Read the model definition and answer for the solid it produces. Units are mm, in the model's axes. A direction names the side the tool comes from. Round coordinates to 2 decimals unless told otherwise and drop trailing zeros. Loops run counter-clockwise (first coordinate to the right, second up) from the corner with the lowest first, then second, coordinate; pieces in that order, holes last. Notation, with made-up numbers: (-33.75, 3) - (-26.75, 3) arc R31 cw to (-26.75, 35) - close; hole circle Ø4 at (49.5, 5.25). An arc over 180 degrees is marked (long way). Use one line per item in the form item = value. Start each with the question number.
```python
from build123d import *

# Parameters (mm, degrees)
PAD028_DEPTH    = 1.4
SKETCH048_R     = 1.75
PAD029_DEPTH    = 1
PAD030_DEPTH    = 1
PAD031_DEPTH    = 1
SKETCH181_W     = 1.5
SKETCH181_H     = 1.5
POCKET062_DEPTH = 1


with BuildPart() as part:
    # Sketch047 (on Face725 of Binder021) → Pad028 (new body)
    with BuildSketch(Plane(origin=(0, 135.8, 0), x_dir=(-1, 0, 0), z_dir=(0, 1, 0))):
        with BuildLine():
            Line((-120.499982, -0.1), (-120.499982, -26.3))
            Line((-120.499982, -26.3), (-68.48194, -26.3))
            ThreePointArc((-67.46705, -26.3), (-67.974495, -21.15), (-68.48194, -26.3))
            Line((-67.46705, -26.3), (-32.299995, -26.3))
            Line((-32.299995, -15.934266), (-32.299995, -26.3))
            ThreePointArc((-31.615729, -15.25), (-32.099578, -15.450417), (-32.299995, -15.934266))
            Line((-31.615729, -15.25), (-23.784261, -15.25))
            ThreePointArc((-23.099995, -15.934266), (-23.300412, -15.450417), (-23.784261, -15.25))
            Line((-23.099995, -15.934266), (-23.099995, -26.3))
            Line((-7.299995, -26.3), (-23.099995, -26.3))
            Line((-7.299995, -26.3), (-7.299995, -0.1))
            Line((-7.299995, -0.1), (-120.499982, -0.1))
        make_face()
        with BuildLine():
            Line((-105.199995, -19.86), (-92.199994, -19.86))
            ThreePointArc((-90.899995, -21.16), (-91.280756, -20.240762), (-92.199994, -19.86))
            Line((-90.899995, -21.16), (-90.899995, -24.776619))
            Line((-90.899995, -24.776619), (-91.938732, -25.120886))
            Line((-91.938732, -25.120886), (-92.869018, -25.773985))
            ThreePointArc((-93.61597, -26.01), (-93.224294, -25.949593), (-92.869018, -25.773985))
            Line((-93.61597, -26.01), (-103.78402, -26.01))
            ThreePointArc((-104.530977, -25.773981), (-104.175699, -25.949592), (-103.78402, -26.01))
            Line((-105.461258, -25.120886), (-104.530977, -25.773981))
            Line((-106.499995, -24.776619), (-105.461258, -25.120886))
            Line((-106.499995, -21.16), (-106.499995, -24.776619))
            ThreePointArc((-105.199995, -19.86), (-106.119234, -20.240761), (-106.499995, -21.16))
        make_face(mode=Mode.SUBTRACT)
    extrude(amount=-PAD028_DEPTH)

    # Sketch048 (on Face5 of Binder022) → Pad029 (join)
    with BuildSketch(Plane.XY.offset(-26.3)):
        with BuildLine():
            Line((18.199995, 134.4), (8.199995, 134.4))
            Line((8.199995, 134.4), (8.199995, 124.1))
            Line((8.199995, 124.1), (13.199995, 124.1))
            ThreePointArc((13.199995, 124.1), (16.735529, 125.564466), (18.199995, 129.1))
            Line((18.199995, 134.4), (18.199995, 129.1))
        make_face()
        with Locations((13.199995, 129.1)):
            Circle(SKETCH048_R, mode=Mode.SUBTRACT)
        with BuildLine():
            Line((109.449995, 134.4), (119.599982, 134.4))
            Line((119.599982, 134.4), (119.599982, 124.35))
            Line((119.599982, 124.35), (114.449995, 124.35))
            ThreePointArc((109.449995, 129.35), (110.914461, 125.814466), (114.449995, 124.35))
            Line((109.449995, 134.4), (109.449995, 129.35))
        make_face()
        with Locations((114.449995, 129.35)):
            Circle(SKETCH048_R, mode=Mode.SUBTRACT)
    extrude(amount=PAD029_DEPTH)

    # Sketch049 (on Face25 of Pad029) → Pad030 (join)
    with BuildSketch(Plane(origin=(8.199995, 0, 0), x_dir=(0, -1, 0), z_dir=(-1, 0, 0))):
        Polygon((-134.4, -25.3), (-124.1, -25.3), (-134.4, -15), align=None)
    extrude(amount=-PAD030_DEPTH)

    # Sketch050 (on Face36 of Pad030) → Pad031 (join)
    with BuildSketch(Plane.YZ.offset(119.599982)):
        Polygon((124.35, -25.3), (134.4, -25.3), (134.4, -15.25), align=None)
    extrude(amount=-PAD031_DEPTH)

    # Sketch181 (on Face5 of Clone006) → Pocket062 (cut)
    with BuildSketch(Plane.XZ.offset(-134.4)):
        with Locations((38.579995, -25.55)):
            Rectangle(SKETCH181_W, SKETCH181_H)
    extrude(amount=-POCKET062_DEPTH, mode=Mode.SUBTRACT)


solid = part.part
```
1) Straight lines are drawn through the part: line 1 (X direction, y = 129.1, z = -25.45); line 2 (X direction, y = 129.35, z = -26); line 3 (Z direction, x = 110, y = 131.5). For each, find the intervals that lie inside material, in ascending order. Write a range as from..to.
2) A cutting plane is placed at A-A on z = -17.25. Write down the section's boundary in (x, y), plus the area to 3 significant figures.
3) A cutting plane is placed at D-D on z = -4.5. Write down the section's boundary in (x, y), plus the area to 3 significant figures.
4) For faces 5 (the flat face through (119.11, 129.45, -20.2)), 6 (the cylindrical face through (110.88, 125.85, -25.81)), 7 (the flat face through (15, 130, -25.3)), 8 (the flat face through (119.6, 130, -22)), determine the directions among +Z, -Z, +X, -X, +Y, -Y from which every point of the face is accessible in a straight line to the end or side of a thin tool.
5) A cutting plane is placed at C-C on x = 53. Write down the section's boundary in (y, z), plus the area to 3 significant figures.
6) Determine the mould class of faces 1 (the flat face through (65, 135.8, -13)), 2 (the cylindrical face through (113.06, 128.29, -25.81)), 3 (the cylindrical face through (12.82, 127.39, -25.81)), 4 (the flat face through (9.2, 132, -22)) for opening direction Y: +Y half, -Y half, draft (parallel to the pull), parting line (faces both ways), or undercut.
7) Flat-ended cylindrical pins translate along their axes: pin 1 (1.1 mm diameter, centred on y = 131, z = -25.5, fed in from +X); pin 2 (5 mm diameter, centred on y = 127, z = -18.5, fed in from +X); pin 3 (8 mm diameter, centred on x = 69, z = -12.5, fed in from -Y). Find the tip coordinate at first contact, or state that the pin passes through.
8) A cutting plane is placed at B-B on z = -23.75. Write down the section's boundary in (x, y), plus the area to 3 significant figures.
Checks:
q1.line_1 = 8.2..11.45, 14.95..18.2, 109.46..112.72, 116.18..119.6
q1.line_2 = 8.2..11.47, 14.93..18.2, 109.45..112.7, 116.2..119.6
q1.line_3 = -26.3..-25.3
q2.outline = (7.3, 134.4) - (8.2, 134.4) - (8.2, 132.15) - (9.2, 132.15) - (9.2, 134.4) - (23.1, 134.4) - (23.1, 135.8) - (7.3, 135.8) - close; (32.3, 134.4) - (118.6, 134.4) - (118.6, 132.4) - (119.6, 132.4) - (119.6, 134.4) - (120.5, 134.4) - (120.5, 135.8) - (32.3, 135.8) - close
q2.area = 150 mm²
q3.outline = (7.3, 134.4) - (120.5, 134.4) - (120.5, 135.8) - (7.3, 135.8) - close
q3.area = 158 mm²
q4.face_5 = +Z, +X, -Y
q4.face_6 = +Z, -Z, -Y
q4.face_7 = +Z, -Y
q4.face_8 = +Z, -Z, +X, -Y
q5.outline = (134.4, -26.3) - (135.8, -26.3) - (135.8, -0.1) - (134.4, -0.1) - close
q5.area = 36.7 mm²
q6.face_1 = +Y half
q6.face_2 = undercut
q6.face_3 = undercut
q6.face_4 = draft
q7.pin_1 = 119.6
q7.pin_2 = through
q7.pin_3 = 134.4
q8.outline = (7.3, 134.4) - (8.2, 134.4) - (8.2, 125.65) - (9.2, 125.65) - (9.2, 134.4) - (23.1, 134.4) - (23.1, 135.8) - (7.3, 135.8) - close; (32.3, 134.4) - (65.37, 134.4) - (65.37, 135.8) - (32.3, 135.8) - close; (70.57, 134.4) - (90.9, 134.4) - (90.9, 135.8) - (70.57, 135.8) - close; (106.5, 134.4) - (118.6, 134.4) - (118.6, 125.9) - (119.6, 125.9) - (119.6, 134.4) - (120.5, 134.4) - (120.5, 135.8) - (106.5, 135.8) - close
q8.area = 134 mm²
